Work out the finished part from the listing and answer in its coordinate system (mm). A direction names the side the tool comes from. Round coordinates to 2 decimals unless told otherwise and drop trailing zeros. Write each loop counter-clockwise with the first axis right and the second up, starting at its lowest first coordinate (ties: lowest second). Pieces come first, ordered by that corner, then holes.
from build123d import *

# Parameters (mm, degrees)
ESQUISSE1_W             = 320
ESQUISSE1_H             = 120
ESQUISSE1_R             = 16
ESQUISSE1_R_2           = 15
ESQUISSE1_R_3           = 2
BOSS_EXTRU_1_DEPTH      = 11
ESQUISSE2_R             = 2.1
ENL_V_MAT_EXTRU_1_DEPTH = 11
ESQUISSE3_OUTSIDE_W     = 390.388
ESQUISSE3_OUTSIDE_H     = 190.388
ENL_V_MAT_EXTRU_2_DEPTH = 268.05991837
CONG_1_R                = 20
ESQUISSE4_R             = 1.8
ENL_V_MAT_EXTRU_3_DEPTH = 262.095767871
ESQUISSE5_R             = 1.8
ENL_V_MAT_EXTRU_4_DEPTH = 262.095767871


with BuildPart() as part:
    # Esquisse1 → Boss.-Extru.1 (new body)
    with BuildSketch(Plane.XY):
        with Locations((-100, 0)):
            Rectangle(ESQUISSE1_W, ESQUISSE1_H)
        Circle(ESQUISSE1_R, mode=Mode.SUBTRACT)
        with Locations((-200, 0)):
            Circle(ESQUISSE1_R_2, mode=Mode.SUBTRACT)
        with Locations((-200, 20)):
            Circle(ESQUISSE1_R_3, mode=Mode.SUBTRACT)
        with Locations((-180, 0)):
            Circle(ESQUISSE1_R_3, mode=Mode.SUBTRACT)
        with Locations((-200, -20)):
            Circle(ESQUISSE1_R_3, mode=Mode.SUBTRACT)
        with Locations((-220, 0)):
            Circle(ESQUISSE1_R_3, mode=Mode.SUBTRACT)
    extrude(amount=BOSS_EXTRU_1_DEPTH)

    # Esquisse2 → Enlèv. mat.-Extru.1 (cut)
    with BuildSketch(Plane.XY.offset(11)):
        with Locations((-200, 25)):
            Circle(ESQUISSE2_R)
        with Locations((-182.32233047, 17.67766953)):
            Circle(ESQUISSE2_R)
        with Locations((-175, 0)):
            Circle(ESQUISSE2_R)
        with Locations((-182.32233047, -17.67766953)):
            Circle(ESQUISSE2_R)
        with Locations((-200, -25)):
            Circle(ESQUISSE2_R)
        with Locations((-217.67766953, -17.67766953)):
            Circle(ESQUISSE2_R)
        with Locations((-225, 0)):
            Circle(ESQUISSE2_R)
        with Locations((-217.67766953, 17.67766953)):
            Circle(ESQUISSE2_R)
        with Locations((0, 25)):
            Circle(ESQUISSE2_R)
        with Locations((17.67766953, 17.67766953)):
            Circle(ESQUISSE2_R)
        with Locations((25, 0)):
            Circle(ESQUISSE2_R)
        with Locations((17.67766953, -17.67766953)):
            Circle(ESQUISSE2_R)
        with Locations((0, -25)):
            Circle(ESQUISSE2_R)
        with Locations((-17.67766953, -17.67766953)):
            Circle(ESQUISSE2_R)
        with Locations((-25, 0)):
            Circle(ESQUISSE2_R)
        with Locations((-17.67766953, 17.67766953)):
            Circle(ESQUISSE2_R)
    extrude(amount=-ENL_V_MAT_EXTRU_1_DEPTH, mode=Mode.SUBTRACT)

    # Esquisse3 outside → Enlèv. mat.-Extru.2 (cut, through all)
    with BuildSketch(Plane.XY.offset(11)):
        with Locations((-100, 0)):
            Rectangle(ESQUISSE3_OUTSIDE_W, ESQUISSE3_OUTSIDE_H)
        with BuildLine():
            Line((-153.902277714, 30), (-46.097722286, 30))
            ThreePointArc((-46.097722286, 30), (55, 0), (-46.097722286, -30))
            Line((-46.097722286, -30), (-153.902277714, -30))
            ThreePointArc((-153.902277714, -30), (-255, 0), (-153.902277714, 30))
        make_face(mode=Mode.SUBTRACT)
    extrude(amount=-ENL_V_MAT_EXTRU_2_DEPTH, mode=Mode.SUBTRACT)

    # Congé1
    cong_1_edges = [part.edges().sort_by_distance(p)[0] for p in [
        (-153.902277714, 30, 5.5),
        (-46.097722286, 30, 5.5),
        (-46.097722286, -30, 5.5),
        (-153.902277714, -30, 5.5),
    ]]
    fillet(cong_1_edges, radius=CONG_1_R)

    # Esquisse4 → Enlèv. mat.-Extru.3 (cut, through all)
    with BuildSketch(Plane.XY.offset(11)):
        with Locations((-200, 51.5)):
            Circle(ESQUISSE4_R)
        with Locations((-169.729059507, 41.66437521)):
            Circle(ESQUISSE4_R)
        with Locations((-151.020589411, 15.91437521)):
            Circle(ESQUISSE4_R)
        with Locations((-151.020589411, -15.91437521)):
            Circle(ESQUISSE4_R)
        with Locations((-169.729059507, -41.66437521)):
            Circle(ESQUISSE4_R)
        with Locations((-200, -51.5)):
            Circle(ESQUISSE4_R)
        with Locations((-230.270940493, -41.66437521)):
            Circle(ESQUISSE4_R)
        with Locations((-248.979410589, -15.91437521)):
            Circle(ESQUISSE4_R)
        with Locations((-248.979410589, 15.91437521)):
            Circle(ESQUISSE4_R)
        with Locations((-230.270940493, 41.66437521)):
            Circle(ESQUISSE4_R)
        with Locations(Location((30.270940493, 41.66437521, 0), (0, 0, 180))):
            Circle(ESQUISSE4_R)
        with Locations(Location((48.979410589, 15.91437521, 0), (0, 0, 180))):
            Circle(ESQUISSE4_R)
        with Locations(Location((48.979410589, -15.91437521, 0), (0, 0, 180))):
            Circle(ESQUISSE4_R)
        with Locations(Location((30.270940493, -41.66437521, 0), (0, 0, 180))):
            Circle(ESQUISSE4_R)
        with Locations(Location((0, -51.5, 0), (0, 0, 180))):
            Circle(ESQUISSE4_R)
        with Locations(Location((-30.270940493, -41.66437521, 0), (0, 0, 180))):
            Circle(ESQUISSE4_R)
        with Locations(Location((-48.979410589, -15.91437521, 0), (0, 0, 180))):
            Circle(ESQUISSE4_R)
        with Locations(Location((-48.979410589, 15.91437521, 0), (0, 0, 180))):
            Circle(ESQUISSE4_R)
        with Locations(Location((-30.270940493, 41.66437521, 0), (0, 0, 180))):
            Circle(ESQUISSE4_R)
        with Locations(Location((0, 51.5, 0), (0, 0, 180))):
            Circle(ESQUISSE4_R)
    extrude(amount=-ENL_V_MAT_EXTRU_3_DEPTH, mode=Mode.SUBTRACT)

    # Esquisse5 → Enlèv. mat.-Extru.4 (cut, through all)
    with BuildSketch(Plane.XY.offset(11)):
        with Locations((-100, 20)):
            Circle(ESQUISSE5_R)
        with Locations((-100, -20)):
            Circle(ESQUISSE5_R)
    extrude(amount=-ENL_V_MAT_EXTRU_4_DEPTH, mode=Mode.SUBTRACT)


solid = part.part
Q1. Find section B-B (x = -92.5). Determine the outline of the cut face in (y, z).
Q2. Find section A-A (y = 9). Determine the outline of the cut face in (x, z), plus the area to 3 significant figures.
Q3. Given pin 1 (1.5 mm diameter, centred on y = 10.5, z = 7, fed in from +X); pin 2 (5 mm diameter, centred on x = 25, y = 0, fed in from +Z); pin 3 (6 mm diameter, centred on x = -98, z = 1.5, fed in from +Y); pin 4 (2 mm diameter, centred on x = -127, z = 7.5, fed in from -Y), each flat-ended and moving along its own axis, determine where each tip first touches the part or whether it passes through.
Q4. Find the intervals of material crossed by L1, parallel to X at y = -4, z = 10; L2, parallel to X at y = -9, z = 9.75; L3, parallel to Y at x = -80.5, z = 3.75, in increasing order.
Q5. A tool of negligible diameter and unlimited length cuts with its end or side. For faces 1 (the face through (-214.985, 0.66, 5.423)), 2 (the face through (-152.156, -31.695, 5.423)), 3 (the face through (-101, 30, 6)), from which of +Z, -Z, +X, -X, +Y, -Y can it reach the whole face along a straight path? Write none if from no direction.
Q6. The mould has two halves that part along X. Classify faces 4 (the face through (-254.97, -1.86, 5.58)), 5 (the face through (-102, 1, 0)): +X half, -X half, draft (parallel to the pull), parting line (faces both ways), or undercut.
Q7. Find section C-C (z = 6.75). Count the separate pieces of the cut face and the enclosed holes in it, plus the area to 3 significant figures.
Report:
1. outline: (-30, 0) - (30, 0) - (30, 11) - (-30, 11) - close
2. outline: (-254.26, 0) - (-212, 0) - (-212, 11) - (-254.26, 11) - close; (-188, 0) - (-13.23, 0) - (-13.23, 11) - (-188, 11) - close; (13.23, 0) - (54.26, 0) - (54.26, 11) - (13.23, 11) - close
2. area: 2,840 mm2
3. pin 1: stops at x = 54.13
3. pin 2: stops at z = 11
3. pin 3: stops at y = 30
3. pin 4: stops at y = -30
4. L1: x = -254.85 to -214.46, -185.54 to -15.49, 15.49 to 54.85
4. L2: x = -254.26 to -212, -188 to -13.23, 13.23 to 54.26
4. L3: y = -30 to 30
5. face 1: +Z, -Z
5. face 2: +Z, -Z, -Y
5. face 3: +Z, -Z, +Y
6. face 4: undercut
6. face 5: draft
7. separate pieces: 1
7. enclosed holes: 44
7. area: 22,800 mm2
